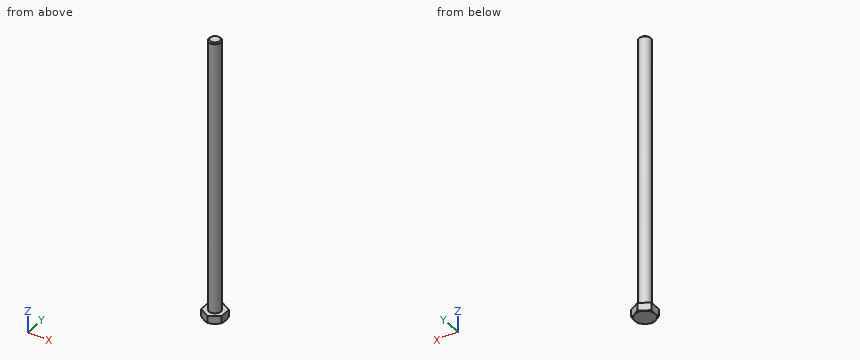
from build123d import *

# Parameters (mm, degrees)
ESQUISSE1_W        = 3
ESQUISSE1_H        = 135
BOSS_EXTRU_1_DEPTH = 4


with BuildPart() as part:
    # Esquisse1 → Base-Révolution (revolve)
    with BuildSketch(Plane(origin=(0, 0, 0), x_dir=(1, 0, 0), z_dir=(0, 1, 0))):
        with Locations((1.5, -67.5)):
            Rectangle(ESQUISSE1_W, ESQUISSE1_H)
    revolve(axis=Axis((0, 0, 0), (0, 0, 1)))

    # Chanfrein1: read off the stored shape, not the designer's step
    # Chanfrein1 outline → Chanfrein1 (revolve, cut)
    with BuildSketch(Plane.XZ):
        Polygon((3, 135), (2.4, 135), (3, 134.4), align=None)
    revolve(axis=Axis((0, 0, 0), (0, 0, 1)), mode=Mode.SUBTRACT)

    # Esquisse6 → Boss.-Extru.1 (add)
    with BuildSketch(Plane.XY):
        Polygon((5, -2.886751346), (5, 2.886751346), (0, 5.773502692), (-5, 2.886751346), (-5, -2.886751346), (0, -5.773502692), align=None)
    extrude(amount=-BOSS_EXTRU_1_DEPTH)

    # Esquisse7 → Enlèvement de matière-Révolution1 (revolve, cut)
    with BuildSketch(Plane(origin=(0, 0, 0), x_dir=(1, 0, 0), z_dir=(0, 1, 0))):
        Polygon((-5, 4), (-11.92820323, 4), (-11.92820323, 0), align=None)
    revolve(axis=Axis((0, 0, -6.239446496), (0, 0, 1)), mode=Mode.SUBTRACT)


solid = part.part
Geometry check sheet. Reference: the model listing, model coordinates, mm. Round coordinates to 2 decimals unless told otherwise and drop trailing zeros. Write each loop counter-clockwise with the first axis right and the second up, starting at its lowest first coordinate (ties: lowest second). Pieces come first, ordered by that corner, then holes.
Item 1: Section check A-A (z = 95.5). Record the boundary of the cut face in (x, y), plus the area to 3 significant figures.
Determined:
outline: circle Ø6 at (0, 0)
area: 28.3 mm2
Item 2: Material ranges on line 1 along Z through (x, y) = (4, 0); line 2 along X through (y, z) = (0.75, 16); line 3 along X through (y, z) = (0.25, 10), recorded low to high.
Determined:
line 1: z = -4 to 0
line 2: x = -2.9 to 2.9
line 3: x = -2.99 to 2.99
Item 3: Go/stop test with flat-tipped pins: pin 1 Ø6 at (y, z) = (4.5, 26) entering from -X; pin 2 Ø5 at (y, z) = (-0.5, 15) entering from +X; pin 3 Ø5 at (x, z) = (0, 48.5) entering from -Y. Record where each tip stops, or that it passes through.
Determined:
pin 1: stops at x = -2.6
pin 2: stops at x = 3
pin 3: stops at y = -3
